from build123d import *

# Parameters (mm, degrees)
SKETCH1_W          = 5
SKETCH1_H          = 12
SKETCH2_R          = 2
CUT_EXTRUDE1_DEPTH = 30
CIRPATTERN1_COUNT  = 8


with BuildPart() as part:
    # Sketch1 → Revolve1 (revolve)
    with BuildSketch(Plane.XY, mode=Mode.PRIVATE) as revolve1_sk:
        with Locations((-83.5, 88.5)):
            Rectangle(SKETCH1_W, SKETCH1_H)
    revolve(revolve1_sk.sketch.rotate(Axis((-206.017932179, 0, 0), (1, 0, 0)), 90), axis=Axis((-206.017932179, 0, 0), (1, 0, 0)))

    # Sketch2 → Cut-Extrude1 (cut)
    with BuildSketch(Plane.ZY.offset(86)):
        with Locations((0, 89.5)):
            Circle(SKETCH2_R)
    cut_extrude1 = extrude(amount=-CUT_EXTRUDE1_DEPTH, mode=Mode.SUBTRACT)

    # CirPattern1: Cut-Extrude1 ×8 about axis
    cirpattern1_axis = Axis((0, 0, 0), (1, 0, 0))
    for i in range(1, CIRPATTERN1_COUNT):
        add(cut_extrude1.rotate(cirpattern1_axis, i * 360 / CIRPATTERN1_COUNT), mode=Mode.SUBTRACT)


solid = part.part
Here's how the part is built. I have some questions about the finished solid (model axes, mm). Round coordinates to 2 decimals unless told otherwise and drop trailing zeros. Loops run counter-clockwise (first coordinate to the right, second up) from the corner with the lowest first, then second, coordinate; pieces in that order, holes last. Notation, with made-up numbers: M -12.75,45.25 L 27.25,45.25 A22 ccw 27.25,77.25 Z; hole C 74,0.5 d6. An arc over 180 degrees is marked long. Write each question's results on one line, items separated by ' | '. Start each with the question number.
(1) Will these pins go through, and if not, where does the flat tip stop? P1, Ø3, axis at x = -83, y = -65, coming from the -Z side; P2, Ø1, axis at x = -83, y = 37, coming from the -Z side; P3, Ø2, axis at x = -83.5, z = -64, coming from the -Y side.
(2) If I drill on probe 1 along Y at (x, z) = (-82.25, 0); probe 2 along Z at (x, y) = (-82.95, -62); probe 3 along Z at (x, y) = (-82.6, -63), over which ranges is the centre line in solid material (lowest first)? Write a range as from..to.
(3) I want a section at A-A (z = -23.5). Please give me the cut outline in (x, y).
(4) I want a section at C-C (x = -83.6). State how many separate pieces and enclosed holes the cut face has, then the cut area to 3 significant figures.
(5) Thinking about a two-plate mould opening in Y: for faces 1 (the cylindrical face through (-83.46, 80.54, -17.88)), 2 (the flat face through (-86, 84, 0)), 3 (the cylindrical face through (-83.46, 92.25, -20.49)), which applies, pulls with the +Y half, pulls with the -Y half, needs draft (parallel to the pull), parting line crosses it, or undercut?
(6) I want a section at B-B (y = 10.5). Please give me the cut outline in (x, z), then the cut area to 3 significant figures.
Solved:
1) P1: stops at z = -69.99 | P2: stops at z = -87.17 | P3: stops at y = -70.44
2) probe 1: y = -94.5..-91.5, -87.5..-82.5, 82.5..87.5, 91.5..94.5 | probe 2: z = -71.32..-64.82, -61.75..-54.43, 54.43..61.75, 64.82..71.32 | probe 3: z = -70.44..-65.27, -61.31..-53.27, 53.27..61.31, 65.27..70.44
3) outline: M -86,-91.53 L -81,-91.53 L -81,-79.08 L -86,-79.08 Z; M -86,79.08 L -81,79.08 L -81,91.53 L -86,91.53 Z
4) separate pieces: 1 | enclosed holes: 9 | area: 6,570 mm²
5) face 1: undercut | face 2: needs draft | face 3: parting line crosses it
6) outline: M -86,-93.91 L -81,-93.91 L -81,-81.83 L -86,-81.83 Z; M -86,81.83 L -81,81.83 L -81,93.91 L -86,93.91 Z | area: 121 mm²
